```python
from build123d import *

# Parameters (mm, degrees)
BOSS_EXTRUDE1_DEPTH      = 19
BOSS_EXTRUDE1_DEPTH_BACK = 19
BOSS_EXTRUDE2_DEPTH      = 9
BOSS_EXTRUDE2_DEPTH_BACK = 9
SKETCH2_W                = 24
SKETCH2_H                = 5
CUT_EXTRUDE2_DEPTH       = 76


with BuildPart() as part:
    # Sketch1 → Boss-Extrude1 (new, two sides: drawn at the far end of the back side and taken through both)
    with BuildSketch(Plane.XY.offset(-BOSS_EXTRUDE1_DEPTH_BACK)):
        Polygon((-35.570076419, -4.126221996), (-1.570076419, 22.873778004), (19.429923581, 22.873778004), (19.429923581, -29.126221996), (-35.570076419, -29.126221996), align=None)
    extrude(amount=BOSS_EXTRUDE1_DEPTH + BOSS_EXTRUDE1_DEPTH_BACK)

    # Sketch1_3 → Boss-Extrude2 (add, two sides: drawn at the far end of the back side and taken through both)
    with BuildSketch(Plane.XY.offset(-BOSS_EXTRUDE2_DEPTH_BACK)):
        Polygon((-55.570076419, -29.126221996), (-35.570076419, -29.126221996), (-35.570076419, -4.126221996), (-16.681187531, 10.873778004), (-55.570076419, 10.873778004), align=None)
    extrude(amount=BOSS_EXTRUDE2_DEPTH + BOSS_EXTRUDE2_DEPTH_BACK)

    # Sketch2 → Cut-Extrude2 (cut)
    with BuildSketch(Plane(origin=(19.429923581, 0, 0), x_dir=(0, 0, -1), z_dir=(1, 0, 0))):
        with Locations((0, 20.373778004)):
            Rectangle(SKETCH2_W, SKETCH2_H)
    extrude(amount=-CUT_EXTRUDE2_DEPTH, mode=Mode.SUBTRACT)


solid = part.part
```
Verification items for the finished model (mm, model axes). A direction names the side the tool comes from. Give positions to 0.01 mm unless a question says otherwise; leave off trailing zeros. Order: outer loops, then holes, each group sorted by start corner. A loop starts at its lowest first (then second) coordinate and runs counter-clockwise, first axis right, second up. Notation, with made-up numbers: (44, 57.25) -> (53, 57.25) arc R26 ccw to (53, 80.25) -> close; hole circle Ø4 at (26, 76.5). An arc over 180 degrees is marked (long way). Use a Markdown table: item, result.
1) Section check D-D, the plane z = 2. Record the boundary of the cut face in (x, y).
Results:
| item | result |
|---|---|
| outline | (-55.57, -29.13) -> (19.43, -29.13) -> (19.43, 17.87) -> (-7.87, 17.87) -> (-16.68, 10.87) -> (-55.57, 10.87) -> close |
2) Section check A-A, the plane x = 5. Record the boundary of the cut face in (y, z).
Results:
| item | result |
|---|---|
| outline | (-29.13, -19) -> (22.87, -19) -> (22.87, -12) -> (17.87, -12) -> (17.87, 12) -> (22.87, 12) -> (22.87, 19) -> (-29.13, 19) -> close |
3) Mould release check, pull along Z, two halves, no side actions. Record for faces 5 (the flat face through (19.43, -3, 0)), 6 (the flat face through (6, 17.874, 0)), 7 (the flat face through (-8, -9, 19)): pulls with the +Z half, pulls with the -Z half, needs draft (parallel to the pull), parting line crosses it, or undercut.
Results:
| item | result |
|---|---|
| face 5 | needs draft |
| face 6 | undercut |
| face 7 | pulls with the +Z half |
4) Section check C-C, the plane z = -10.5. Record the boundary of the cut face in (x, y).
Results:
| item | result |
|---|---|
| outline | (-35.57, -29.13) -> (19.43, -29.13) -> (19.43, 17.87) -> (-7.87, 17.87) -> (-35.57, -4.13) -> close |
5) Section check B-B, the plane y = -24. Record the boundary of the cut face in (x, z).
Results:
| item | result |
|---|---|
| outline | (-55.57, -9) -> (-35.57, -9) -> (-35.57, -19) -> (19.43, -19) -> (19.43, 19) -> (-35.57, 19) -> (-35.57, 9) -> (-55.57, 9) -> close |
6) Material ranges on probe 1 along Z at (x, y) = (8, 20); probe 2 along X at (y, z) = (-9, 14.5); probe 3 along Y at (x, z) = (13, -9), recorded low to high.
Results:
| item | result |
|---|---|
| probe 1 | -19 to -12, 12 to 19 |
| probe 2 | -35.57 to 19.43 |
| probe 3 | -29.13 to 17.87 |
7) Depth check by flat-ended pin: pin 1 Ø19 at (x, z) = (5, -4) entering from +Y; pin 2 Ø8 at (x, z) = (-15, -13) entering from +Y; pin 3 Ø11.5 at (x, y) = (-43, -4.5) entering from -Z; pin 4 Ø5.5 at (x, z) = (-30.5, 1.5) entering from +Y. Enter the tip coordinate at first touch or a pass-through.
Results:
| item | result |
|---|---|
| pin 1 | y = 22.87 |
| pin 2 | y = 15.39 |
| pin 3 | z = -9 |
| pin 4 | y = 10.87 |
8) Tool access check on faces 1 (the flat face through (-36, 10.874, 0)), 2 (the flat face through (-35.57, -17, -14)), 3 (the flat face through (6, 20, 12)), 4 (the flat face through (-35.57, -17, 14)). Record the directions out of +Z, -Z, +X, -X, +Y, -Y that give a thin tool (end or side, any length) a straight path to the whole face; none if there is none.
Results:
| item | result |
|---|---|
| face 1 | +Z, -Z, -X, +Y |
| face 2 | -Z, -X, +Y, -Y |
| face 3 | +X, -X, +Y |
| face 4 | +Z, -X, +Y, -Y |
